Geometry check sheet. Reference: the model listing, model coordinates, mm. A direction names the side the tool comes from. Coordinates: 2 decimals unless noted, no trailing zeros. Write each loop counter-clockwise with the first axis right and the second up, starting at its lowest first coordinate (ties: lowest second). Pieces come first, ordered by that corner, then holes. Notation, with made-up numbers: (23, 41) -> (70, 41) arc R26 ccw to (70, 57) -> close; hole circle Ø11 at (11.5, 75.5). An arc over 180 degrees is marked (long way). Answer in a Markdown table with one row per item. Add a question column.
1. Depth check by flat-ended pin: P1, Ø2, axis at y = 10, z = -0.5, coming from the +X side; P2, Ø0.7, axis at x = -0.5, z = 0.5, coming from the -Y side; P3, Ø3, axis at x = 2, y = 10.5, coming from the -Z side. Enter the tip coordinate at first touch or a pass-through.
2. Scan lines: L1, parallel to X at y = 2.45, z = 0; L2, parallel to X at y = 1.5, z = 0.5; L3, parallel to Y at x = 0.5, z = -1. Record each from-to range of solid material in increasing order. Write a range as from..to.
3. Cross-section at C-C on y = 2.5. Record the cut outline in (x, z), and give its area (3 significant figures).
4. Cross-section at D-D on x = 3.25. Record the cut outline in (y, z).
5. Cross-section at A-A on x = 0. Record the cut outline in (y, z) (3 decimals).
6. Mould release check, pull along Z, two halves, no side actions. Record for faces 1 (the cylindrical face through (-1.01, 2.96, -0.65)), 2 (the cylindrical face through (-3.417, 10.423, -0.759)), 3 (the flat face through (-2, 5, 2)): pulls with the +Z half, pulls with the -Z half, needs draft (parallel to the pull), parting line crosses it, or undercut.
7. Cross-section at B-B on z = 0. Record the cut outline in (x, y) (3 decimals), and give its area (3 significant figures).
8. Set-up check for faces 4 (the flat face through (0, 16, 0)), 5 (the cylindrical face through (-2.44, 2.46, -0.54)): record each of +Z, -Z, +X, -X, +Y, -Y from which the full face is reachable in a straight line by a thin tool's end or side.
```python
from build123d import *

# Parameters (mm, degrees)
SKETCH1_R           = 2.5
BOSS_EXTRUDE1_DEPTH = 5
SKETCH2_R           = 3.5
BOSS_EXTRUDE2_DEPTH = 11


with BuildPart() as part:
    # Sketch1 → Boss-Extrude1 (new body)
    with BuildSketch(Plane(origin=(0, 0, 0), x_dir=(1, 0, 0), z_dir=(0, 1, 0))):
        with Locations(Location((0, 0, 0), (0, 0, 270))):
            Circle(SKETCH1_R)
    extrude(amount=BOSS_EXTRUDE1_DEPTH)

    # Sketch7 → CSK for M2 Oval Head Machine Screw2 (revolve, cut)
    with BuildSketch(Plane(origin=(0, 0, 0), x_dir=(0, 0, -1), z_dir=(1, 0, 0))):
        Polygon((0, 0), (0, 5), (1.225, 5), (1.2, 4.975), (1.2, 1), (2.2, 0), align=None)
    revolve(axis=Axis((0, -6.35, 0), (0, 1, 0)), mode=Mode.SUBTRACT)

    # Sketch2 → Boss-Extrude2 (add)
    with BuildSketch(Plane(origin=(0, 5, 0), x_dir=(1, 0, 0), z_dir=(0, 1, 0))):
        with Locations(Location((0, 0, 0), (0, 0, 270))):
            Circle(SKETCH2_R)
    extrude(amount=BOSS_EXTRUDE2_DEPTH)


solid = part.part
```
Results found:
| question | item | result |
|---|---|---|
| 1 | P1 | stops at x = 3.5 |
| 1 | P2 | stops at y = 5 |
| 1 | P3 | stops at z = -3.46 |
| 2 | L1 | x = -2.5..-1.2, 1.2..2.5 |
| 2 | L2 | x = -2.45..-1.09, 1.09..2.45 |
| 2 | L3 | y = 5..16 |
| 3 | outline | circle Ø5 at (0, 0); hole circle Ø2.4 at (0, 0) |
| 3 | area | 15.1 mm^2 |
| 4 | outline | (5, -1.3) -> (16, -1.3) -> (16, 1.3) -> (5, 1.3) -> close |
| 5 | outline | (0, -2.5) -> (5, -2.5) -> (5, -3.5) -> (16, -3.5) -> (16, 3.5) -> (5, 3.5) -> (5, 2.5) -> (0, 2.5) -> (0, 2.2) -> (1, 1.2) -> (4.975, 1.2) -> (5, 1.225) -> (5, -1.225) -> (4.975, -1.2) -> (1, -1.2) -> (0, -2.2) -> close |
| 6 | face 1 | undercut |
| 6 | face 2 | parting line crosses it |
| 6 | face 3 | needs draft |
| 7 | outline | (-3.5, 5) -> (-2.5, 5) -> (-2.5, 0) -> (-2.2, 0) -> (-1.2, 1) -> (-1.2, 4.975) -> (-1.225, 5) -> (1.225, 5) -> (1.2, 4.975) -> (1.2, 1) -> (2.2, 0) -> (2.5, 0) -> (2.5, 5) -> (3.5, 5) -> (3.5, 16) -> (-3.5, 16) -> close |
| 7 | area | 89.0 mm^2 |
| 8 | face 4 | +Z, -Z, +X, -X, +Y |
| 8 | face 5 | -Y |
